```python
from build123d import *

# Parameters (mm, degrees)
ESQUISSE1_R                  = 8
ESQUISSE1_R_2                = 1.5
EXTRUSION1_DEPTH             = 12
EXTRUSION2_DEPTH             = 17.492422502
R_P_TITION_CIRCULAIRE1_COUNT = 18
ESQUISSE3_R                  = 10
ESQUISSE3_R_2                = 5.6
EXTRUSION3_DEPTH             = 1
R_P_TITION_LIN_AIRE1_COUNT   = 2
R_P_TITION_LIN_AIRE1_PITCH   = 13


with BuildPart() as part:
    # Esquisse1 → Extrusion1 (new body)
    with BuildSketch(Plane.XY):
        Circle(ESQUISSE1_R)
        Circle(ESQUISSE1_R_2, mode=Mode.SUBTRACT)
    extrude(amount=EXTRUSION1_DEPTH)

    # Esquisse2 → Extrusion2 (cut, through all)
    with BuildSketch(Plane.XY.offset(12)):
        Polygon((-0.6, 7.353512063), (0.6, 7.353512063), (1.002277566, 8.216199086), (-1.002277566, 8.216199086), align=None)
    extrusion2 = extrude(amount=-EXTRUSION2_DEPTH, mode=Mode.SUBTRACT)

    # Répétition circulaire1: Extrusion2 ×18 about axis
    r_p_tition_circulaire1_axis = Axis((0, 0, 0), (0, 0, 1))
    for i in range(1, R_P_TITION_CIRCULAIRE1_COUNT):
        add(extrusion2.rotate(r_p_tition_circulaire1_axis, i * 360 / R_P_TITION_CIRCULAIRE1_COUNT), mode=Mode.SUBTRACT)

    # Esquisse3 → Extrusion3 (add)
    with BuildSketch(Plane.XY.offset(12)):
        Circle(ESQUISSE3_R)
        Circle(ESQUISSE3_R_2, mode=Mode.SUBTRACT)
    extrusion3 = extrude(amount=EXTRUSION3_DEPTH)

    # Répétition linéaire1: Extrusion3 ×2
    with Locations(*[(0, 0, -i * R_P_TITION_LIN_AIRE1_PITCH) for i in range(1, R_P_TITION_LIN_AIRE1_COUNT)]):
        add(extrusion3)


solid = part.part
```
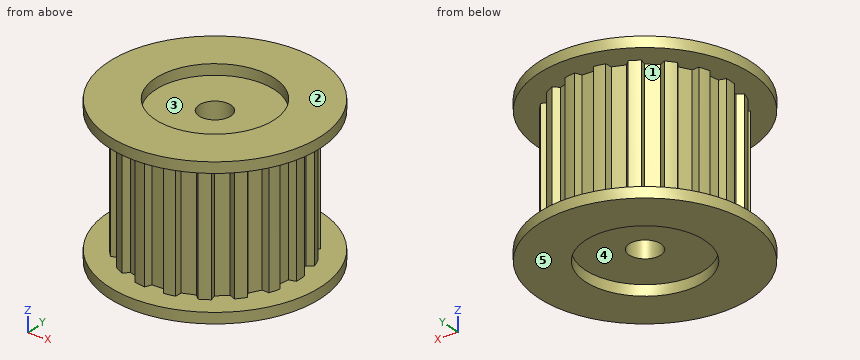
Can you work these out from the model? Positions are in its coordinate system, mm. Face numbers are marked on the shaded views. A direction names the side the tool comes from. Round coordinates to 2 decimals unless told otherwise and drop trailing zeros. Loops run counter-clockwise (first coordinate to the right, second up) from the corner with the lowest first, then second, coordinate; pieces in that order, holes last. Notation, with made-up numbers: M -3.5,89.5 L 18.5,89.5 A19 ccw 18.5,108.5 Z; hole C 75,39.25 d5. An arc over 180 degrees is marked long. Answer as a JSON object with one key per item and string values. Group by question number.
Q1. We'd pull the mould along Y, two halves only. Please class the marked faces 4 and 5: +Y half, -Y half, draft (parallel to the pull), parting line (faces both ways), or undercut.
Q2. On a 3-axis mill with a long thin cutter (end or side, diameter ignored), from which of +Z, -Z, +X, -X, +Y, -Y can I reach the whole of each face in a straight line? I mean the marked faces 1, 2 and 3. Say none if no direction works.
Q3. Please list where these lines run through material, in increasing order: L1, parallel to Z at x = 0.25, y = 7.75; L2, parallel to Y at x = 0, z = 9; L3, parallel to Y at x = 0, z = -0.2.
Q4. Imagine slicing it at B-B, the plane x = 0. Please give me the cut outline in (y, z).
Q5. Imagine slicing it at A-A, the plane y = 0. Please give me the cut outline in (x, z).
Q6. Will these pins go through, and if not, where does the flat tip stop? pin 1 (6 mm diameter, centred on x = -0.5, y = -0.5, fed in from -Z); pin 2 (9 mm diameter, centred on x = 0, y = 0, fed in from +Z); pin 3 (5 mm diameter, centred on x = -6.5, z = 8, fed in from -Y).
Q7. Imagine slicing it at D-D, the plane x = -4. Please give me the cut outline in (y, z).
Q8. Imagine slicing it at C-C, the plane x = 2.5. Please give me the cut outline in (y, z), then the cut area to 3 significant figures.
Findings:
{
 "1": {"face 4": "undercut", "face 5": "draft"},
 "2": {"face 1": "none", "face 2": "+Z, +X, -X, +Y, -Y", "face 3": "+Z"},
 "3": {"L1": "z = -1 to 0, 12 to 13", "L2": "y = -7.35 to -1.5, 1.5 to 7.35", "L3": "y = -10 to -5.6, 5.6 to 10"},
 "4": {"outline": "M -10,-1 L -5.6,-1 L -5.6,0 L -1.5,0 L -1.5,12 L -5.6,12 L -5.6,13 L -10,13 L -10,12 L -7.35,12 L -7.35,0 L -10,0 Z; M 1.5,0 L 5.6,0 L 5.6,-1 L 10,-1 L 10,0 L 7.35,0 L 7.35,12 L 10,12 L 10,13 L 5.6,13 L 5.6,12 L 1.5,12 Z"},
 "5": {"outline": "M -10,-1 L -5.6,-1 L -5.6,0 L -1.5,0 L -1.5,12 L -5.6,12 L -5.6,13 L -10,13 L -10,12 L -8,12 L -8,0 L -10,0 Z; M 1.5,0 L 5.6,0 L 5.6,-1 L 10,-1 L 10,0 L 8,0 L 8,12 L 10,12 L 10,13 L 5.6,13 L 5.6,12 L 1.5,12 Z"},
 "6": {"pin 1": "stops at z = 0", "pin 2": "stops at z = 12", "pin 3": "stops at y = -6.93"},
 "7": {"outline": "M -9.17,-1 L -3.92,-1 L -3.92,0 L 3.92,0 L 3.92,-1 L 9.17,-1 L 9.17,0 L 6.93,0 L 6.93,12 L 9.17,12 L 9.17,13 L 3.92,13 L 3.92,12 L -3.92,12 L -3.92,13 L -9.17,13 L -9.17,12 L -6.93,12 L -6.93,0 L -9.17,0 Z"},
 "8": {"outline": "M -9.68,-1 L -5.01,-1 L -5.01,0 L 5.01,0 L 5.01,-1 L 9.68,-1 L 9.68,0 L 6.92,0 L 6.92,12 L 9.68,12 L 9.68,13 L 5.01,13 L 5.01,12 L -5.01,12 L -5.01,13 L -9.68,13 L -9.68,12 L -6.92,12 L -6.92,0 L -9.68,0 Z", "area": "185 mm2"}
}
